```python
from build123d import *

# Parameters (mm, degrees)
SKETCH_W        = 50
SKETCH_H        = 35
SKETCH_R        = 6.5
PAD_DEPTH       = 25
SKETCH001_R     = 13.15
POCKET_DEPTH    = 16
SKETCH002_R     = 2.6
POCKET001_DEPTH = 35.001


with BuildPart() as part:
    # Sketch → Pad (new body)
    with BuildSketch(Plane.XY):
        with Locations((0, 0.5)):
            Rectangle(SKETCH_W, SKETCH_H)
        Circle(SKETCH_R, mode=Mode.SUBTRACT)
    extrude(amount=PAD_DEPTH)

    # Sketch001 (on Face7 of Pad) → Pocket (cut)
    with BuildSketch(Plane.XY.offset(25)):
        Circle(SKETCH001_R)
    extrude(amount=-POCKET_DEPTH, mode=Mode.SUBTRACT)

    # Sketch002 (on Face1 of Pocket) → Pocket001 (cut, through all)
    with BuildSketch(Plane(origin=(0, 18, 0), x_dir=(-1, 0, 0), z_dir=(0, 1, 0))):
        with Locations((-16, 6)):
            Circle(SKETCH002_R)
        with Locations((16, 6)):
            Circle(SKETCH002_R)
        with Locations((-16, 18)):
            Circle(SKETCH002_R)
        with Locations((16, 18)):
            Circle(SKETCH002_R)
    extrude(amount=-POCKET001_DEPTH, mode=Mode.SUBTRACT)


solid = part.part
```
Source: CAD feature listing. Evaluate the final solid. Frame: model axes, mm. A direction names the side the tool comes from. Round coordinates to 2 decimals unless told otherwise and drop trailing zeros. Loops run counter-clockwise (first coordinate to the right, second up) from the corner with the lowest first, then second, coordinate; pieces in that order, holes last.
(1) Material intervals for probe 1 along Z at (x, y) = (-16, 0.5); probe 2 along Y at (x, z) = (0, 2.25); probe 3 along Z at (x, y) = (15, -5), sorted ascending.
From the geometry:
probe 1: z = 0 to 3.4, 8.6 to 15.4, 20.6 to 25
probe 2: y = -17 to -6.5, 6.5 to 18
probe 3: z = 0 to 3.6, 8.4 to 15.6, 20.4 to 25
(2) Section query A-A (z = 6). Output: boundary loops of the cut face in (x, y).
From the geometry:
outline: (-25, -17) - (-18.6, -17) - (-18.6, 18) - (-25, 18) - close; (-13.4, -17) - (13.4, -17) - (13.4, 18) - (-13.4, 18) - close; (18.6, -17) - (25, -17) - (25, 18) - (18.6, 18) - close; hole circle Ø13 at (0, 0)
(3) Access query for faces 4 (the cylindrical face through (-13.137, 0.578, 17.112)), 5 (the cylindrical face through (-18.48, 0.75, 6.78)). Directions: +Z, -Z, +X, -X, +Y, -Y. A direction counts if a zero-diameter tool reaches every point of the face in a straight line with its end or side. Return the directions, or none.
From the geometry:
face 4: +Z
face 5: +Y, -Y
(4) Contact query for flat-ended pins moving along their axis: pin 1 Ø4.5 at (x, z) = (-16, 6) entering from +Y; pin 2 Ø1 at (x, y) = (-15.5, 8) entering from -Z. Output: stop coordinate, or through.
From the geometry:
pin 1: passes through
pin 2: stops at z = 0
(5) Pull-direction query (Y, two-part tool) for faces 1 (the flat face through (-6, -3, 9)), 2 (the flat face through (-6, 5, 0)), 3 (the flat face through (0, 18, 12)); classes: +Y half, -Y half, draft (parallel to the pull), parting line (faces both ways), or undercut.
From the geometry:
face 1: undercut
face 2: draft
face 3: +Y half
(6) Section query B-B (y = 0). Output: boundary loops of the cut face in (x, z), and give its area (3 significant figures).
From the geometry:
outline: (-25, 0) - (-6.5, 0) - (-6.5, 9) - (-13.15, 9) - (-13.15, 25) - (-25, 25) - close; (6.5, 0) - (25, 0) - (25, 25) - (13.15, 25) - (13.15, 9) - (6.5, 9) - close; hole circle Ø5.2 at (-16, 6); hole circle Ø5.2 at (-16, 18); hole circle Ø5.2 at (16, 6); hole circle Ø5.2 at (16, 18)
area: 627 mm2
(7) Section query D-D (x = -1). Output: boundary loops of the cut face in (y, z), and give its area (3 significant figures).
From the geometry:
outline: (-17, 0) - (-6.42, 0) - (-6.42, 9) - (-13.11, 9) - (-13.11, 25) - (-17, 25) - close; (6.42, 0) - (18, 0) - (18, 25) - (13.11, 25) - (13.11, 9) - (6.42, 9) - close
area: 340 mm2
(8) Section query C-C (x = -16). Output: boundary loops of the cut face in (y, z).
From the geometry:
outline: (-17, 0) - (18, 0) - (18, 3.4) - (-17, 3.4) - close; (-17, 8.6) - (18, 8.6) - (18, 15.4) - (-17, 15.4) - close; (-17, 20.6) - (18, 20.6) - (18, 25) - (-17, 25) - close
